The model under review builds one solid part; all positions refer to its coordinate system, in mm. Give positions to 0.01 mm unless a question says otherwise; leave off trailing zeros. Loops run counter-clockwise (first coordinate to the right, second up) from the corner with the lowest first, then second, coordinate; pieces in that order, holes last. Notation, with made-up numbers: (78.25, -25.75) - (132.25, -25.75) arc R35 ccw to (132.25, 11.25) - close; hole circle Ø10 at (54, 88.5). An arc over 180 degrees is marked (long way). Return JSON: item names as keys, results as strings. Group by question number.
Autodesk Inventor part; units mm, degrees
ref_plane "YZ Plane" through (0, 0, 0) normal (1, 0, 0) x (0, 1, 0)
ref_plane "XZ Plane" through (0, 0, 0) normal (0, 1, 0) x (-1, 0, 0)
ref_plane "XY Plane" through (0, 0, 0) normal (0, 0, 1) x (1, 0, 0)
sketch "スケッチ1" plane through (0, 0, 0) normal (0, 1, 0) x (-1, 0, 0)
  circle A0 centre (0, 0) radius 14
  dimension "d0" = 28
extrude "押し出し1" add sketch "スケッチ1" along normal blind 0.5
sketch "スケッチ2" plane through (0, 0.5, 0) normal (0, 1, 0) x (1, 0, 0)
  circle A0 centre (0, -11) radius 1.7
  circle A1 centre (9.5263, 5.5) radius 1.7
  circle A2 centre (-9.5263, 5.5) radius 1.7
  point P0 (0, 0)
  dimension "d4" = 3.4
  dimension "d12" = 11
  dimension "d15" = 360
extrude "押し出し2" cut sketch "スケッチ2" against normal through all
sketch "スケッチ3" plane through (0, 0.5, 0) normal (0, 1, 0) x (1, 0, 0)
  circle A0 centre (0, 0) radius 5
  dimension "d9" = 10
extrude "押し出し3" cut sketch "スケッチ3" against normal through all
properties part number "B_holder_up_5" material "ステンレス鋼 440C"
1) We need section C-C, the plane z = 11. Write out the cut boundary in (x, y), plus the area to 3 significant figures.
2) We need section D-D, the plane z = -5.5. Write out the cut boundary in (x, y).
3) We need section A-A, the plane x = 0. Write out the cut boundary in (y, z), plus the area to 3 significant figures.
4) To check wall thickness, follow line 1 (Z direction, x = 0, y = 0.25); line 2 (X direction, y = 0.1, z = -5.5); line 3 (X direction, y = 0.35, z = -0.75). State the ranges of each line that lie inside material, in increasing order.
5) We need section B-B, the plane y = 0.1. Write out the cut boundary in (x, z).
6) Draft analysis for pull direction Z (two halves, no side actions). For faces 1 (the face through (-0.37, 0.25, 12.66)), 2 (the face through (-12.932, 0.246, 5.362)), 3 (the face through (0, 0.5, -6)), state which applies: +Z half, -Z half, draft (parallel to the pull), parting line (faces both ways), or undercut.
Findings:
{
 "1": {"outline": "(-8.66, 0) - (-1.7, 0) - (-1.7, 0.5) - (-8.66, 0.5) - close; (1.7, 0) - (8.66, 0) - (8.66, 0.5) - (1.7, 0.5) - close", "area": "6.96 mm^2"},
 "2": {"outline": "(-12.87, 0) - (-11.23, 0) - (-11.23, 0.5) - (-12.87, 0.5) - close; (-7.83, 0) - (7.83, 0) - (7.83, 0.5) - (-7.83, 0.5) - close; (11.23, 0) - (12.87, 0) - (12.87, 0.5) - (11.23, 0.5) - close"},
 "3": {"outline": "(0, -14) - (0.5, -14) - (0.5, -5) - (0, -5) - close; (0, 5) - (0.5, 5) - (0.5, 9.3) - (0, 9.3) - close; (0, 12.7) - (0.5, 12.7) - (0.5, 14) - (0, 14) - close", "area": "7.30 mm^2"},
 "4": {"line 1": "z = -14 to -5, 5 to 9.3, 12.7 to 14", "line 2": "x = -12.87 to -11.23, -7.83 to 7.83, 11.23 to 12.87", "line 3": "x = -13.98 to -4.94, 4.94 to 13.98"},
 "5": {"outline": "circle Ø28 at (0, 0); hole circle Ø3.4 at (-9.53, -5.5); hole circle Ø10 at (0, 0); hole circle Ø3.4 at (0, 11); hole circle Ø3.4 at (9.53, -5.5)"},
 "6": {"face 1": "undercut", "face 2": "parting line", "face 3": "draft"}
}
